Part model, mm, in its own coordinate system. Face numbers are marked on the shaded views. A direction names the side the tool comes from. Coordinates: 2 decimals unless noted, no trailing zeros. Loops run counter-clockwise (first coordinate to the right, second up) from the corner with the lowest first, then second, coordinate; pieces in that order, holes last. Notation, with made-up numbers: (50, 84) -> (60, 84) arc R29 cw to (60, 116) -> close; hole circle Ø6 at (-7.5, 55). An arc over 180 degrees is marked (long way). Use one line per item in the form item = value. Start each with the question number.
(1) Pin check, flat tips, straight feed: P1, Ø1, axis at y = -2, z = -6.5, coming from the -X side; P2, Ø1, axis at x = 25, y = 17.5, coming from the -Z side; P3, Ø2, axis at x = 24, y = -10.5, coming from the -Z side; P4, Ø2.5, axis at x = 24, y = -2.5, coming from the +Z side. Stop position of each tip, or through.
(2) Mould opens along Y. For the marked faces 1, 2, 3 and 4 say: +Y half, -Y half, draft (parallel to the pull), parting line (faces both ways), or undercut.
(3) Band-saw the part on A-A on x = 35. Give the cut face in (y, z), then the cut area to 3 significant figures.
(4) Band-saw the part on B-B on y = -1. Give the cut face in (x, z).
(5) Band-saw the part on C-C on z = -10. Give the cut face in (x, y).
(6) 3-axis set-ups, long thin cutter, end or side, ignore diameter. For the marked faces 5 and 6: which of +Z, -Z, +X, -X, +Y, -Y reach the whole face in a straight line?
(7) Band-saw the part on D-D on y = -31. Give the cut face in (x, z).
(8) Drill centre lines: L1, parallel to Y at x = 5, z = -8; L2, parallel to Y at x = 29.5, z = -11.75; L3, parallel to X at y = -30, z = -12. Where is each one in solid material? Low to high. Write a range as [from, to].
```python
from build123d import *

# Parameters (mm, degrees)
BOSS_EXTRUDE1_DEPTH = 36
CUT_EXTRUDE1_DEPTH  = 16.5
SKETCH3_W           = 8
SKETCH3_H           = 77.131502371
CUT_EXTRUDE2_DEPTH  = 0.6
SKETCH4_R           = 2.6
CUT_EXTRUDE3_DEPTH  = 56.865910894


with BuildPart() as part:
    # Sketch1 → Boss-Extrude1 (new, symmetric)
    with BuildSketch(Plane(origin=(0, 0, 0), x_dir=(1, 0, 0), z_dir=(0, 1, 0))):
        with BuildLine():
            Line((27.5, 15), (40, 15))
            Line((40, 15), (40, 0))
            Line((40, 0), (0, 0))
            Line((0, 0), (0, 15))
            Line((0, 15), (12.5, 15))
            ThreePointArc((12.5, 15), (20, 7.5), (27.5, 15))
        make_face()
    extrude(amount=BOSS_EXTRUDE1_DEPTH, both=True)

    # Sketch2 → Cut-Extrude1 (cut, symmetric)
    with BuildSketch(Plane(origin=(0, 0, 0), x_dir=(1, 0, 0), z_dir=(0, 1, 0))):
        with BuildLine():
            Line((8.458861594, 15), (31.458861594, 15))
            ThreePointArc((31.458861594, 15), (19.958861594, 3.5), (8.458861594, 15))
        make_face()
    extrude(amount=CUT_EXTRUDE1_DEPTH, both=True, mode=Mode.SUBTRACT)

    # Sketch3 → Cut-Extrude2 (cut)
    with BuildSketch(Plane.XY):
        with Locations((22.8, -0.239836761)):
            Rectangle(SKETCH3_W, SKETCH3_H)
    extrude(amount=-CUT_EXTRUDE2_DEPTH, mode=Mode.SUBTRACT)

    # Sketch4 → Cut-Extrude3 (cut, through all)
    with BuildSketch(Plane.XY):
        with Locations((5, 31)):
            Circle(SKETCH4_R)
        with Locations((35, 31)):
            Circle(SKETCH4_R)
        with Locations((35, -31)):
            Circle(SKETCH4_R)
        with Locations((5, -31)):
            Circle(SKETCH4_R)
        with Locations((35, 0)):
            Circle(SKETCH4_R)
    extrude(amount=-CUT_EXTRUDE3_DEPTH, mode=Mode.SUBTRACT)


solid = part.part
```
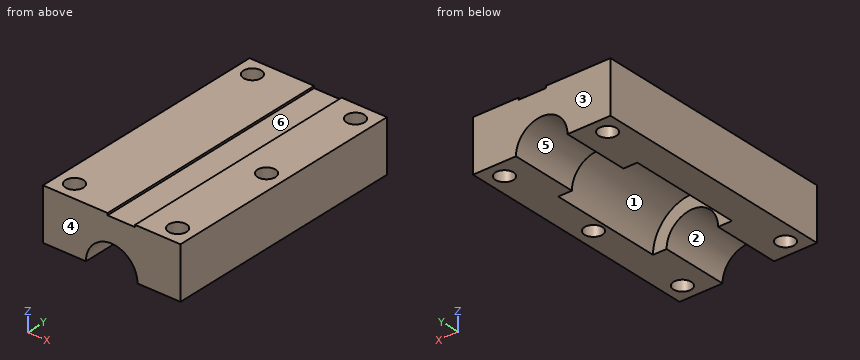
A:
q1.P1 = 0
q1.P2 = -9.9
q1.P3 = -4.66
q1.P4 = -0.6
q2.face_1 = undercut
q2.face_2 = draft
q2.face_3 = +Y half
q2.face_4 = -Y half
q3.outline = (-36, -15) -> (-33.6, -15) -> (-33.6, 0) -> (-36, 0) -> close; (-28.4, -15) -> (-2.6, -15) -> (-2.6, 0) -> (-28.4, 0) -> close; (2.6, -15) -> (28.4, -15) -> (28.4, 0) -> (2.6, 0) -> close; (33.6, -15) -> (36, -15) -> (36, 0) -> (33.6, 0) -> close
q3.area = 846 mm²
q4.outline = (0, -15) -> (8.46, -15) arc R11.5 cw to (31.46, -15) -> (32.6, -15) -> (32.6, 0) -> (26.8, 0) -> (26.8, -0.6) -> (18.8, -0.6) -> (18.8, 0) -> (0, 0) -> close; (37.4, -15) -> (40, -15) -> (40, 0) -> (37.4, 0) -> close
q5.outline = (0, -36) -> (14.41, -36) -> (14.41, -16.5) -> (9.6, -16.5) -> (9.6, 16.5) -> (14.41, 16.5) -> (14.41, 36) -> (0, 36) -> close; (25.59, -36) -> (40, -36) -> (40, 36) -> (25.59, 36) -> (25.59, 16.5) -> (30.32, 16.5) -> (30.32, -16.5) -> (25.59, -16.5) -> close; hole circle Ø5.2 at (5, -31); hole circle Ø5.2 at (5, 31); hole circle Ø5.2 at (35, -31); hole circle Ø5.2 at (35, 0); hole circle Ø5.2 at (35, 31)
q6.face_5 = -Z, +Y, -Y
q6.face_6 = +Z, +Y, -Y
q7.outline = (0, -15) -> (2.4, -15) -> (2.4, 0) -> (0, 0) -> close; (7.6, -15) -> (12.5, -15) arc R7.5 cw to (27.5, -15) -> (32.4, -15) -> (32.4, 0) -> (26.8, 0) -> (26.8, -0.6) -> (18.8, -0.6) -> (18.8, 0) -> (7.6, 0) -> close; (37.6, -15) -> (40, -15) -> (40, 0) -> (37.6, 0) -> close
q8.L1 = [-36, -33.6], [-28.4, 28.4], [33.6, 36]
q8.L2 = [-36, -16.5], [16.5, 36]
q8.L3 = [0, 2.6], [7.4, 13.13], [26.87, 32.6], [37.4, 40]
